from build123d import *

# Parameters (mm, degrees)
SKETCH1_W           = 7.0575
SKETCH1_H           = 97
BOSS_EXTRUDE2_DEPTH = 7.6
SKETCH4_W           = 5
SKETCH4_H           = 91.05
CUT_EXTRUDE1_DEPTH  = 4.85
SKETCH6_W           = 5
SKETCH6_H           = 91.05
BOSS_EXTRUDE3_DEPTH = 2.75
SKETCH8_W           = 7.0575
SKETCH8_H           = 97
BOSS_EXTRUDE4_DEPTH = 1
SKETCH9_W           = 5
SKETCH9_H           = 11
BOSS_EXTRUDE5_DEPTH = 6.5
CUT_EXTRUDE2_DEPTH  = 2.4
SKETCH11_R          = 1.85
CUT_EXTRUDE3_DEPTH  = 50.293805962
FILLET2_R           = 5


with BuildPart() as part:
    # Sketch1 → Boss-Extrude2 (new body)
    with BuildSketch(Plane(origin=(0, 0, 0), x_dir=(1, 0, 0), z_dir=(0, 1, 0))):
        Rectangle(SKETCH1_W, SKETCH1_H)
    extrude(amount=BOSS_EXTRUDE2_DEPTH)

    # Sketch4 → Cut-Extrude1 (cut)
    with BuildSketch(Plane(origin=(0, 7.6, 0), x_dir=(1, 0, 0), z_dir=(0, 1, 0))):
        with Locations((1.02875, -2.975)):
            Rectangle(SKETCH4_W, SKETCH4_H)
    extrude(amount=-CUT_EXTRUDE1_DEPTH, mode=Mode.SUBTRACT)

    # Sketch6 → Boss-Extrude3 (add)
    with BuildSketch(Plane(origin=(0, 7.6, 0), x_dir=(1, 0, 0), z_dir=(0, 1, 0))):
        with Locations((1.02875, -2.975)):
            Rectangle(SKETCH6_W, SKETCH6_H)
    extrude(amount=-BOSS_EXTRUDE3_DEPTH)

    # Sketch8 → Boss-Extrude4 (add)
    with BuildSketch(Plane.XZ):
        Rectangle(SKETCH8_W, SKETCH8_H)
    extrude(amount=BOSS_EXTRUDE4_DEPTH)

    # Sketch9 → Boss-Extrude5 (add)
    with BuildSketch(Plane.XZ.offset(1)):
        with Locations((-1.02875, 43)):
            Rectangle(SKETCH9_W, SKETCH9_H)
        with Locations((-1.02875, -43)):
            Rectangle(SKETCH9_W, SKETCH9_H)
    extrude(amount=BOSS_EXTRUDE5_DEPTH)

    # Sketch10 → Cut-Extrude2 (cut)
    with BuildSketch(Plane(origin=(1.47125, 0, 0), x_dir=(0, 0, -1), z_dir=(1, 0, 0))):
        Polygon((-44.58771324, -0.75), (-46.175426481, -3.5), (-44.58771324, -6.25), (-41.41228676, -6.25), (-39.824573519, -3.5), (-41.41228676, -0.75), align=None)
        Polygon((46.175426481, -3.5), (44.58771324, -0.75), (41.41228676, -0.75), (39.824573519, -3.5), (41.41228676, -6.25), (44.58771324, -6.25), align=None)
    extrude(amount=-CUT_EXTRUDE2_DEPTH, mode=Mode.SUBTRACT)

    # Sketch11 → Cut-Extrude3 (cut, through all)
    with BuildSketch(Plane(origin=(-0.92875, 0, 0), x_dir=(0, 0, -1), z_dir=(1, 0, 0))):
        with Locations((-43, -3.5)):
            Circle(SKETCH11_R)
        with Locations((43, -3.5)):
            Circle(SKETCH11_R)
    extrude(amount=-CUT_EXTRUDE3_DEPTH, mode=Mode.SUBTRACT)

    # Fillet2
    fillet2_edges = [part.edges().sort_by_distance(p)[0] for p in [
        (-1.02875, -7.5, 48.5),
        (-1.02875, -7.5, 37.5),
        (-1.02875, -7.5, -37.5),
        (-1.02875, -7.5, -48.5),
    ]]
    fillet(fillet2_edges, radius=FILLET2_R)


solid = part.part
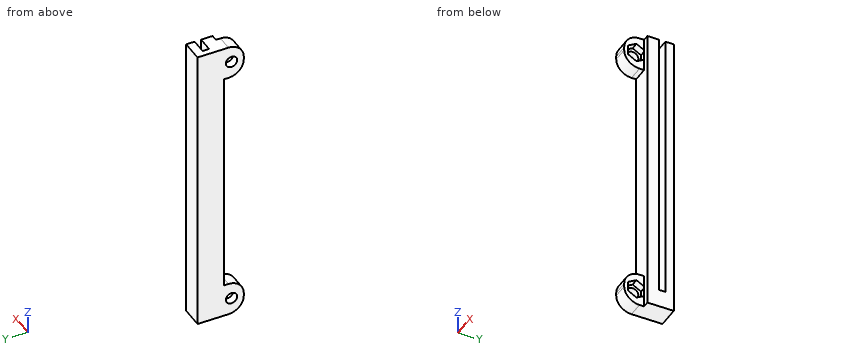
Geometry: final body of the model. Coordinates: model frame, mm. Give positions to 0.01 mm unless a question says otherwise; leave off trailing zeros. Loops run counter-clockwise (first coordinate to the right, second up) from the corner with the lowest first, then second, coordinate; pieces in that order, holes last. Notation, with made-up numbers: (11.5, 33) - (35.5, 33) arc R11 cw to (35.5, 43) - close; hole circle Ø11 at (-27, 83.5). An arc over 180 degrees is marked (long way). One line per question, with ' | ' between items. Start each with the question number.
(1) Section query B-B on z = -27. Return loops of the section in (x, y), then the cut area to 3 significant figures.
(2) Section query A-A on x = 0.5. Return loops of the section in (y, z).
(3) Ray query, line 1 (Y direction, x = -2, z = 43); line 2 (Y direction, x = -1.25, z = -2); line 3 (Y direction, x = -0.5, z = -41.5). Return the intervals inside material, ascending. Write a range as from..to.
(4) Contact query for flat-ended pins moving along their axis: pin 1 (7 mm diameter, centred on y = -5, z = -43, fed in from +X); pin 2 (0.6 mm diameter, centred on x = 0, y = 4, fed in from +Z); pin 3 (3.5 mm diameter, centred on x = -0.5, z = 11, fed in from -Y). Output: stop coordinate, or through.
The answers:
1) outline: (-3.53, -1) - (3.53, -1) - (3.53, 2.75) - (-1.47, 2.75) - (-1.47, 4.85) - (3.53, 4.85) - (3.53, 7.6) - (-3.53, 7.6) - close | area: 50.2 mm2
2) outline: (-7.5, -43.5) arc R5 ccw to (-2.5, -48.5) - (7.6, -48.5) - (7.6, 48.5) - (4.85, 48.5) - (4.85, -42.55) - (2.75, -42.55) - (2.75, 48.5) - (-2.5, 48.5) arc R5 ccw to (-7.5, 43.5) - (-7.5, 42.5) arc R5 ccw to (-2.5, 37.5) - (-1, 37.5) - (-1, -37.5) - (-2.5, -37.5) arc R5 ccw to (-7.5, -42.5) - close; hole (-6.25, -44.59) - (-3.5, -46.18) - (-0.75, -44.59) - (-0.75, -41.41) - (-3.5, -39.82) - (-6.25, -41.41) - close; hole (-6.25, 41.41) - (-3.5, 39.82) - (-0.75, 41.41) - (-0.75, 44.59) - (-3.5, 46.18) - (-6.25, 44.59) - close
3) line 1: -7.5..-5.35, -1.65..7.6 | line 2: -1..2.75, 4.85..7.6 | line 3: -7.4..-6.25, -0.75..2.75, 4.85..7.6
4) pin 1: x = 1.47 | pin 2: z = -42.55 | pin 3: y = -1
